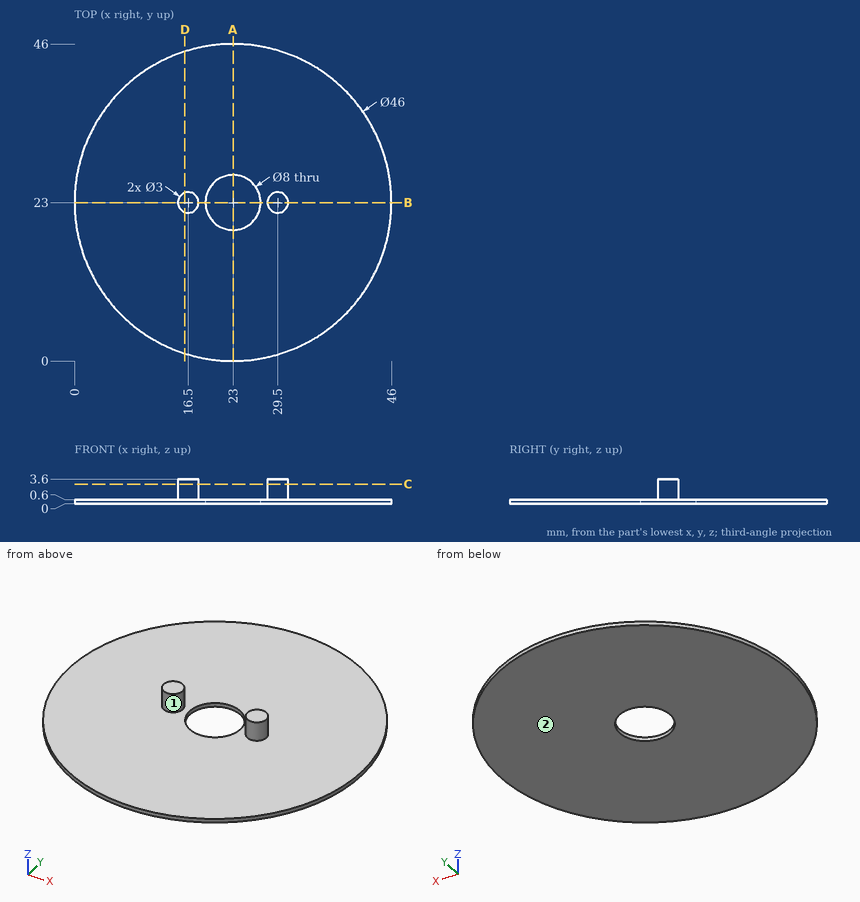
Geometry: see drawing. Coordinates: mm, zero at the bounding-box minimum. Give positions to 0.01 mm unless a question says otherwise; leave off trailing zeros. Write each loop counter-clockwise with the first axis right and the second up, starting at its lowest first coordinate (ties: lowest second). Pieces come first, ordered by that corner, then holes. Notation, with made-up numbers: M -1,26 L 24,26 A16 ccw 24,49 Z; hole C 30,26.25 d11. An arc over 180 degrees is marked long. Answer in a Markdown table with one row per item. Add a question column.
(1) Section A-A on x = 23. Return loops of the section in (y, z).
(2) Section C-C on z = 2.85. Return loops of the section in (x, y).
(3) First-contact query: pin 1 (1 mm diameter, centred on x = 26.5, y = 28, fed in from +Z); pin 2 (1.5 mm diameter, centred on x = 17.5, z = 2.5, fed in from -Y); pin 3 (1.5 mm diameter, centred on x = 11.5, y = 37.5, fed in from -Z). Flat tips, straight axial feed; report the tip coordinate or a pass-through.
(4) Section B-B on y = 23. Return loops of the section in (x, z), and give its area (3 significant figures).
(5) Ray query, line 1 (Y direction, x = 23, z = 0.4); line 2 (Z direction, x = 17, y = 13.5); line 3 (Y direction, x = 17, z = 1.6). Return the intervals inside material, ascending.
(6) Section D-D on x = 16. Return loops of the section in (y, z).
(7) Mould query, pull axis X, two halves, no side actions, for the marked faces 1 and 2. Classes: +X half, -X half, draft (parallel to the pull), parting line (faces both ways), or undercut.
Result set:
| question | item | result |
|---|---|---|
| 1 | outline | M 0,0 L 19,0 L 19,0.6 L 0,0.6 Z; M 27,0 L 46,0 L 46,0.6 L 27,0.6 Z |
| 2 | outline | C 16.5,23 d3; C 29.5,23 d3 |
| 3 | pin 1 | stops at z = 0.6 |
| 3 | pin 2 | stops at y = 21.52 |
| 3 | pin 3 | stops at z = 0 |
| 4 | outline | M 0,0 L 19,0 L 19,0.6 L 18,0.6 L 18,3.6 L 15,3.6 L 15,0.6 L 0,0.6 Z; M 27,0 L 46,0 L 46,0.6 L 31,0.6 L 31,3.6 L 28,3.6 L 28,0.6 L 27,0.6 Z |
| 4 | area | 40.8 mm^2 |
| 5 | line 1 | y = 0 to 19, 27 to 46 |
| 5 | line 2 | z = 0 to 0.6 |
| 5 | line 3 | y = 21.59 to 24.41 |
| 6 | outline | M 1.09,0 L 44.91,0 L 44.91,0.6 L 24.41,0.6 L 24.41,3.6 L 21.59,3.6 L 21.59,0.6 L 1.09,0.6 Z |
| 7 | face 1 | undercut |
| 7 | face 2 | draft |
